```python
from build123d import *

# Parameters (mm, degrees)
SKETCH1_W           = 1105
SKETCH1_H           = 1012.5
SKETCH1_W_2         = 285
SKETCH1_H_2         = 200
SKETCH1_W_3         = 980
SKETCH1_H_3         = 100
BOSS_EXTRUDE1_DEPTH = 1400
SKETCH2_W           = 1105
SKETCH2_H           = 1012.5
BOSS_EXTRUDE3_DEPTH = 62.5
SKETCH3_W           = 980
SKETCH3_H           = 887.5
CUT_EXTRUDE1_DEPTH  = 700
BOSS_EXTRUDE4_REACH = 1107.19
SKETCH5_W           = 980
SKETCH5_H           = 100
SKETCH4_W           = 65
SKETCH4_H           = 10
SKETCH4_W_2         = 60
BOSS_EXTRUDE5_DEPTH = 10
FILLET1_R           = 10
BOSS_EXTRUDE6_START = 62.5
BOSS_EXTRUDE6_DEPTH = 62.5
BOSS_EXTRUDE7_START = -62.5
BOSS_EXTRUDE7_DEPTH = 300
CHAMFER3_SIZE2      = 150
CHAMFER3_SIZE       = 26.449047106
CHAMFER4_SIZE       = 30
CHAMFER4_SIZE_2     = 170.138454589
SKETCH14_W          = 283.550952894
SKETCH14_H          = 180
CUT_EXTRUDE4_DEPTH  = 259


# Some blends are built 0.0001 mm under size
with BuildPart() as part:
    # Sketch1 → Boss-Extrude1 (new body)
    with BuildSketch(Plane.XY):
        with Locations((22.5, 50)):
            Rectangle(SKETCH1_W, SKETCH1_H)
        with Locations((370, 131.25)):
            Rectangle(SKETCH1_W_2, SKETCH1_H_2, mode=Mode.SUBTRACT)
        with Locations((370, 393.75)):
            Rectangle(SKETCH1_W_2, SKETCH1_H_2, mode=Mode.SUBTRACT)
        with Locations((22.5, 393.75)):
            Rectangle(SKETCH1_W_2, SKETCH1_H_2, mode=Mode.SUBTRACT)
        with Locations((-325, 393.75)):
            Rectangle(SKETCH1_W_2, SKETCH1_H_2, mode=Mode.SUBTRACT)
        with Locations((-325, 131.25)):
            Rectangle(SKETCH1_W_2, SKETCH1_H_2, mode=Mode.SUBTRACT)
        with Locations((-325, -131.25)):
            Rectangle(SKETCH1_W_2, SKETCH1_H_2, mode=Mode.SUBTRACT)
        with Locations((22.5, -343.75)):
            Rectangle(SKETCH1_W_3, SKETCH1_H_3, mode=Mode.SUBTRACT)
        with Locations((370, -131.25)):
            Rectangle(SKETCH1_W_2, SKETCH1_H_2, mode=Mode.SUBTRACT)
        with Locations((22.5, -131.25)):
            Rectangle(SKETCH1_W_2, SKETCH1_H_2, mode=Mode.SUBTRACT)
        with Locations((22.5, 131.25)):
            Rectangle(SKETCH1_W_2, SKETCH1_H_2, mode=Mode.SUBTRACT)
    extrude(amount=-BOSS_EXTRUDE1_DEPTH)

    # Sketch2 → Boss-Extrude3 (add)
    with BuildSketch(Plane(origin=(0, 0, -1400), x_dir=(-1, 0, 0), z_dir=(0, 0, -1))):
        with Locations((-22.5, 50)):
            Rectangle(SKETCH2_W, SKETCH2_H)
    extrude(amount=BOSS_EXTRUDE3_DEPTH)

    # Sketch3 → Cut-Extrude1 (cut)
    with BuildSketch(Plane.XY):
        with Locations((22.5, 50)):
            Rectangle(SKETCH3_W, SKETCH3_H)
    extrude(amount=-CUT_EXTRUDE1_DEPTH, mode=Mode.SUBTRACT)

    # Sketch5 → Boss-Extrude4 (add, up to next)
    with BuildSketch(Plane.XY.offset(-700), mode=Mode.PRIVATE) as boss_extrude4_sk1:
        with Locations((22.5, -343.75)):
            Rectangle(SKETCH5_W, SKETCH5_H)
    boss_extrude4_tool1 = extrude(boss_extrude4_sk1.sketch, amount=-BOSS_EXTRUDE4_REACH, mode=Mode.PRIVATE) - part.part
    add(boss_extrude4_tool1.solids().sort_by_distance((22.5, -343.75, -700))[0])

    # Sketch4 → Boss-Extrude5 (add)
    with BuildSketch(Plane.XY.offset(-700)):
        with Locations((-325, 298.75)):
            Rectangle(SKETCH4_W, SKETCH4_H)
        with Locations((-437.5, 298.75)):
            Rectangle(SKETCH4_W_2, SKETCH4_H)
        with Locations((-212.5, 298.75)):
            Rectangle(SKETCH4_W_2, SKETCH4_H)
        with Locations((-90, 298.75)):
            Rectangle(SKETCH4_W_2, SKETCH4_H)
        with Locations((22.5, 298.75)):
            Rectangle(SKETCH4_W, SKETCH4_H)
        with Locations((135, 298.75)):
            Rectangle(SKETCH4_W_2, SKETCH4_H)
        with Locations((257.5, 298.75)):
            Rectangle(SKETCH4_W_2, SKETCH4_H)
        with Locations((370, 298.75)):
            Rectangle(SKETCH4_W, SKETCH4_H)
        with Locations((482.5, 298.75)):
            Rectangle(SKETCH4_W_2, SKETCH4_H)
        with Locations((-437.5, 36.25)):
            Rectangle(SKETCH4_W_2, SKETCH4_H)
        with Locations((-325, 36.25)):
            Rectangle(SKETCH4_W, SKETCH4_H)
        with Locations((-212.5, 36.25)):
            Rectangle(SKETCH4_W_2, SKETCH4_H)
        with Locations((-90, 36.25)):
            Rectangle(SKETCH4_W_2, SKETCH4_H)
        with Locations((22.5, 36.25)):
            Rectangle(SKETCH4_W, SKETCH4_H)
        with Locations((135, 36.25)):
            Rectangle(SKETCH4_W_2, SKETCH4_H)
        with Locations((257.5, 36.25)):
            Rectangle(SKETCH4_W_2, SKETCH4_H)
        with Locations((370, 36.25)):
            Rectangle(SKETCH4_W, SKETCH4_H)
        with Locations((482.5, 36.25)):
            Rectangle(SKETCH4_W_2, SKETCH4_H)
        with Locations((-437.5, -226.25)):
            Rectangle(SKETCH4_W_2, SKETCH4_H)
        with Locations((-325, -226.25)):
            Rectangle(SKETCH4_W, SKETCH4_H)
        with Locations((-212.5, -226.25)):
            Rectangle(SKETCH4_W_2, SKETCH4_H)
        with Locations((-90, -226.25)):
            Rectangle(SKETCH4_W_2, SKETCH4_H)
        with Locations((22.5, -226.25)):
            Rectangle(SKETCH4_W, SKETCH4_H)
        with Locations((135, -226.25)):
            Rectangle(SKETCH4_W_2, SKETCH4_H)
        with Locations((257.5, -226.25)):
            Rectangle(SKETCH4_W_2, SKETCH4_H)
        with Locations((370, -226.25)):
            Rectangle(SKETCH4_W, SKETCH4_H)
        with Locations((482.5, -226.25)):
            Rectangle(SKETCH4_W_2, SKETCH4_H)
    extrude(amount=-BOSS_EXTRUDE5_DEPTH)

    # Fillet1
    fillet1_edges = [part.edges().sort_by_distance(p)[0] for p in [
        (-530, 556.25, -731.25),
        (575, 556.25, -731.25),
    ]]
    fillet(fillet1_edges, radius=FILLET1_R)

    # Sketch6 → Boss-Extrude6 (add)
    with BuildSketch(Plane.XY.offset(BOSS_EXTRUDE6_START)):
        with BuildLine():
            Line((-530, -456.25), (575, -456.25))
            Line((575, -456.25), (575, 546.25))
            ThreePointArc((575, 546.25), (572.071067812, 553.321067812), (565, 556.25))
            Line((565, 556.25), (-520, 556.25))
            ThreePointArc((-520, 556.25), (-527.071067812, 553.321067812), (-530, 546.25))
            Line((-530, 546.25), (-530, -456.25))
        make_face()
    extrude(amount=-BOSS_EXTRUDE6_DEPTH)

    # Sketch8 → Boss-Extrude7 (add)
    with BuildSketch(Plane.ZY.offset(530).offset(BOSS_EXTRUDE7_START)):
        Polygon((62.5, 77.94107028), (212.5, 23.34553514), (212.5, -176.65446486), (62.5, -231.25), align=None)
    extrude(amount=-BOSS_EXTRUDE7_DEPTH)

    # Chamfer3
    chamfer3_edges = [part.edges().sort_by_distance(p)[0] for p in [
        (-167.5, -76.65446486, 62.5),
    ]]
    chamfer3_side = [part.faces().sort_by_distance(p)[0] for p in [
        (-166.971019058, -76.65446486, 62.5),
    ]]
    chamfer(chamfer3_edges, length=CHAMFER3_SIZE - 0.0001, length2=CHAMFER3_SIZE2 - 0.0001, reference=chamfer3_side[0])  # a hair under: the kernel refuses the full size

    # Chamfer4
    # the kernel refuses this chamfer: 170.138454589, 30 mm, written as the material it adds along each edge
    with BuildSketch(Plane(origin=(-467.5, -673.361375011, 62.5), x_dir=(-0.9776715712462578, 0, -0.21013876076743535), z_dir=(0, 1, 0))) as chamfer4_piece_1_section:
        Polygon((CHAMFER4_SIZE * 0.977671571246, CHAMFER4_SIZE * 0.210138760767), (-CHAMFER4_SIZE_2 * 0.210138760767, CHAMFER4_SIZE_2 * 0.977671571244), (0, 0), align=None)
    chamfer4_piece_1 = extrude(amount=1193.413820303, mode=Mode.PRIVATE)
    chamfer4_piece_1 = split(chamfer4_piece_1, bisect_by=Plane(origin=(-476.496724396, -196.562071995, 157.804298923), z_dir=(0, 0.9396926207859072, -0.34202014332567215)), keep=Keep.TOP, mode=Mode.PRIVATE)
    chamfer4_piece_1 = split(chamfer4_piece_1, bisect_by=Plane(origin=(-476.496724396, 43.253142274, 157.804298923), z_dir=(0, -0.9396926207859073, -0.3420201433256722)), keep=Keep.TOP, mode=Mode.PRIVATE)
    chamfer4_piece_1 = split(chamfer4_piece_1, bisect_by=Plane(origin=(-476.496724396, -76.65446486, 212.5), z_dir=(0, 0, -1)), keep=Keep.TOP, mode=Mode.PRIVATE)
    add(chamfer4_piece_1)

    # Sketch14 → Cut-Extrude4 (cut)
    with BuildSketch(Plane.XY.offset(212.5)):
        with Locations((-319.275476447, -76.65446486)):
            Rectangle(SKETCH14_W, SKETCH14_H)
    extrude(amount=-CUT_EXTRUDE4_DEPTH, mode=Mode.SUBTRACT)


solid = part.part
```
Check sheet for the modelled part. Datum: model origin and axes. Units: mm. A direction names the side the tool comes from. Round coordinates to 2 decimals unless told otherwise and drop trailing zeros. Order: outer loops, then holes, each group sorted by start corner. A loop starts at its lowest first (then second) coordinate and runs counter-clockwise, first axis right, second up. Notation, with made-up numbers: (77.5, -29.5) - (94.5, -29.5) arc R25 cw to (94.5, 5.5) - close; hole circle Ø5 at (62, 22). An arc over 180 degrees is marked (long way). Write item = value, one per line.
Q1. Go/stop test with a flat-tipped pin: pin 1 (12 mm diameter, centred on x = -292.5, y = 317, fed in from +Z). Record where the tip stops, or that it passes through.
Computed:
pin_1 = 62.5
Q2. Section check C-C (y = -352.5). Record the boundary of the cut face in (x, z), and give its area (3 significant figures).
Computed:
outline = (-530, -1462.5) - (575, -1462.5) - (575, 62.5) - (-530, 62.5) - close; hole (-467.5, -700) - (512.5, -700) - (512.5, 0) - (-467.5, 0) - close
area = 999,000 mm^2
Q3. Section check B-B (x = 86). Record the boundary of the cut face in (y, z).
Computed:
outline = (-456.25, -1462.5) - (556.25, -1462.5) - (556.25, 62.5) - (-456.25, 62.5) - close; hole (-393.75, -700) - (-231.25, -700) - (-231.25, -1400) - (-31.25, -1400) - (-31.25, -700) - (31.25, -700) - (31.25, -1400) - (231.25, -1400) - (231.25, -700) - (293.75, -700) - (293.75, -1400) - (493.75, -1400) - (493.75, 0) - (-393.75, 0) - close
Q4. Draft check along X on faces 4 (the face through (30, 556.25, -689)), 5 (the face through (-484.46, -78.82, 136.45)), 6 (the face through (-323, -130, -1400)). Enter one of: pulls with the +X half, pulls with the -X half, needs draft (parallel to the pull), parting line crosses it, or undercut.
Computed:
face_4 = needs draft
face_5 = pulls with the -X half
face_6 = undercut
Q5. Thickness scan on line 1 along Y through (x, z) = (-314.5, -755); line 2 along X through (y, z) = (303, -1151.5); line 3 along Z through (x, y) = (19.5, -21.5). Record the ranges inside material, lowest first.
Computed:
line_1 = -456.25 to -231.25, -31.25 to 31.25, 231.25 to 293.75, 493.75 to 556.25
line_2 = -530 to -467.5, -182.5 to -120, 165 to 227.5, 512.5 to 575
line_3 = -1462.5 to -700, 0 to 62.5
Q6. Section check A-A (z = -590.5). Record the boundary of the cut face in (x, y).
Computed:
outline = (-530, -456.25) - (575, -456.25) - (575, 546.25) arc R10 ccw to (565, 556.25) - (-520, 556.25) arc R10 ccw to (-530, 546.25) - close; hole (-467.5, -393.75) - (512.5, -393.75) - (512.5, 493.75) - (-467.5, 493.75) - close
Q7. Tool access check on faces 1 (the face through (-321, 13.346, 108)), 2 (the face through (21, 231.25, -1045)), 3 (the face through (575, 38, -689)). Record the directions out of +Z, -Z, +X, -X, +Y, -Y that give a thin tool (end or side, any length) a straight path to the whole face; none if there is none.
Computed:
face_1 = +Z
face_2 = none
face_3 = +Z, -Z, +X, +Y, -Y
